```python
from build123d import *

# Parameters (mm, degrees)
SKETCH1_R               = 10
SKETCH1_W               = 40
SKETCH1_H               = 8
BOSS_EXTRUDE1_DEPTH     = 12
BOSS_EXTRUDE2_DEPTH     = 19
CUT_EXTRUDE1_DEPTH      = 38
CUT_EXTRUDE1_DEPTH_BACK = 38
SKETCH4_R               = 6
FILLET1_R               = 7
SKETCH6_R               = 6.25
CUT_EXTRUDE2_DEPTH      = 5
CUT_EXTRUDE3_DEPTH      = 56
CUT_EXTRUDE3_DEPTH_BACK = 21
SKETCH9_R               = 5
CUT_EXTRUDE4_DEPTH      = 14
SKETCH10_R              = 5
CUT_EXTRUDE5_DEPTH      = 11


with BuildPart() as part:
    # Sketch1 → Boss-Extrude1 (new, symmetric)
    # profile 1 of 2: a face of its own
    with BuildSketch(Plane.XY):
        Polygon((49.483339502, 12.718271103), (43.983339502, 22.244550544), (0, 30), (-8, 30), (-30.516660498, 17), (-30.516660498, 8), (-30.516660498, 0), (0, 0), (27.454647768, 0), align=None)
        with Locations((-4, 15)):
            Circle(SKETCH1_R, mode=Mode.SUBTRACT)
    # profile 2 of 2: a face of its own
    with BuildSketch(Plane.XY):
        with Locations((-50.516660498, 4)):
            Rectangle(SKETCH1_W, SKETCH1_H)
    extrude(amount=BOSS_EXTRUDE1_DEPTH, both=True)

    # Sketch2 → Boss-Extrude2 (add, symmetric)
    with BuildSketch(Plane.XY):
        Polygon((17.483339502, 26.917215533), (17.483339502, 0), (27.454647768, 0), (49.483339502, 12.718271103), (43.983339502, 22.244550544), align=None)
    extrude(amount=BOSS_EXTRUDE2_DEPTH, both=True)

    # Sketch4 → Cut-Extrude1 (cut, two sides: drawn at the far end of the back side and taken through both)
    with BuildSketch(Plane(origin=(1.363661942, -2.361931768, 0), x_dir=(-0.8660254037844379, -0.5000000000000014, 0), z_dir=(0.5000000000000014, -0.8660254037844379, 0)).offset(-CUT_EXTRUDE1_DEPTH_BACK)):
        with Locations((-31.137235053, 6)):
            Circle(SKETCH4_R)
        with Locations((-38.137235053, -6)):
            Circle(SKETCH4_R)
    extrude(amount=CUT_EXTRUDE1_DEPTH + CUT_EXTRUDE1_DEPTH_BACK, mode=Mode.SUBTRACT)

    # Fillet1
    fillet1_edges = [part.edges().sort_by_distance(p)[0] for p in [
        (17.483339502, 13.458607766, -12),
        (17.483339502, 13.458607766, 12),
    ]]
    fillet(fillet1_edges, radius=FILLET1_R - 0.0001)  # a hair under: the kernel refuses the full size

    # Sketch6 → Cut-Extrude2 (cut)
    with BuildSketch(Plane(origin=(0, 8, 0), x_dir=(1, 0, 0), z_dir=(0, 1, 0))):
        with Locations(Location((-61.516660498, 0, 0), (0, 0, 180))):
            Circle(SKETCH6_R)
    extrude(amount=-CUT_EXTRUDE2_DEPTH, mode=Mode.SUBTRACT)

    # Sketch8 → Cut-Extrude3 (cut, two sides: drawn at the far end of the back side and taken through both)
    with BuildSketch(Plane(origin=(0, 0, 0), x_dir=(0, 0, -1), z_dir=(1, 0, 0)).offset(-CUT_EXTRUDE3_DEPTH_BACK)):
        with BuildLine():
            Line((-9.5, 30), (-2.5, 30))
            ThreePointArc((-2.5, 30), (-6, 26.5), (-9.5, 30))
        make_face()
        with BuildLine():
            Line((2.5, 30), (9.5, 30))
            ThreePointArc((9.5, 30), (6, 26.5), (2.5, 30))
        make_face()
    extrude(amount=CUT_EXTRUDE3_DEPTH + CUT_EXTRUDE3_DEPTH_BACK, mode=Mode.SUBTRACT)

    # Sketch9 → Cut-Extrude4 (cut)
    with BuildSketch(Plane.XY.offset(19)):
        with Locations((34.148109615, 17.12820927)):
            Circle(SKETCH9_R)
    extrude(amount=-CUT_EXTRUDE4_DEPTH, mode=Mode.SUBTRACT)

    # Sketch10 → Cut-Extrude5 (cut)
    with BuildSketch(Plane(origin=(0, 0, -19), x_dir=(-1, 0, 0), z_dir=(0, 0, -1))):
        with Locations((-26.120496882, 17.032442386)):
            Circle(SKETCH10_R)
    extrude(amount=-CUT_EXTRUDE5_DEPTH, mode=Mode.SUBTRACT)


solid = part.part
```
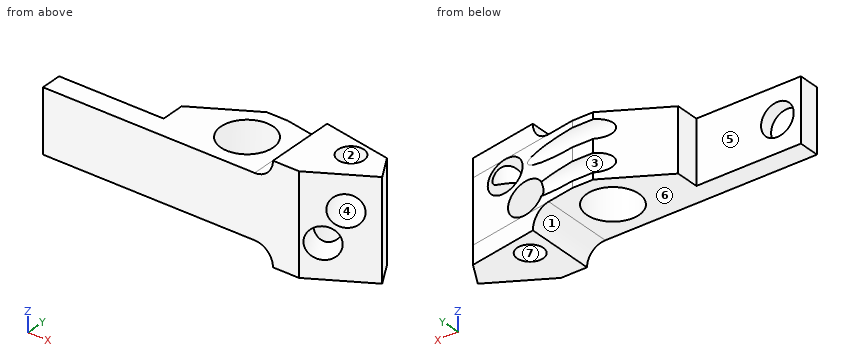
Verification items for the finished model (mm, model axes). Face numbers are marked on the shaded views. A direction names the side the tool comes from. Give positions to 0.01 mm unless a question says otherwise; leave off trailing zeros. Order: outer loops, then holes, each group sorted by start corner. A loop starts at its lowest first (then second) coordinate and runs counter-clockwise, first axis right, second up. Notation, with made-up numbers: (62.5, -36) -> (87.5, -36) arc R33 ccw to (87.5, -2) -> close; hole circle Ø5 at (-16.5, 35.5). An arc over 180 degrees is marked (long way). Use a Markdown table: item, result.
1) Mould release check, pull along Z, two halves, no side actions. Record for the marked faces 1, 2, 3 and 4: pulls with the +Z half, pulls with the -Z half, needs draft (parallel to the pull), parting line crosses it, or undercut.
Results:
| item | result |
|---|---|
| face 1 | pulls with the -Z half |
| face 2 | needs draft |
| face 3 | undercut |
| face 4 | undercut |
2) Section check C-C, the plane x = -59. Record the boundary of the cut face in (y, z).
Results:
| item | result |
|---|---|
| outline | (0, -12) -> (8, -12) -> (8, -5.72) -> (3, -5.72) -> (3, 5.72) -> (8, 5.72) -> (8, 12) -> (0, 12) -> close |
3) Depth check by flat-ended pin: pin 1 Ø12 at (x, y) = (-4, 15) entering from -Z; pin 2 Ø4 at (y, z) = (11.5, -13.5) entering from -X; pin 3 Ø9 at (x, y) = (-32, 20.5) entering from -Z; pin 4 Ø7 at (x, z) = (-56.5, 0.5) entering from +Y. Enter the tip coordinate at first touch or a pass-through.
Results:
| item | result |
|---|---|
| pin 1 | through |
| pin 2 | x = -30.52 |
| pin 3 | z = -12 |
| pin 4 | y = 8 |
4) Tool access check on the marked faces 5, 6 and 7. Record the directions out of +Z, -Z, +X, -X, +Y, -Y that give a thin tool (end or side, any length) a straight path to the whole face; none if there is none.
Results:
| item | result |
|---|---|
| face 5 | +Z, -Z, -X, +Y |
| face 6 | -Z, -X, +Y, -Y |
| face 7 | -Z |
5) Section check A-A, the plane x = -4. Record the boundary of the cut face in (y, z), then the cut area to 3 significant figures.
Results:
| item | result |
|---|---|
| outline | (0, -12) -> (5, -12) -> (5, 12) -> (0, 12) -> close; (25, -12) -> (30, -12) -> (30, -9.5) arc R3.5 cw to (30, -2.5) -> (30, 2.5) arc R3.5 cw to (30, 9.5) -> (30, 12) -> (25, 12) -> close |
| area | 202 mm² |
6) Section check B-B, the plane y = 10.5. Give the number of separate pieces and of enclosed holes in the cut face, then the cut area to 3 significant figures.
Results:
| item | result |
|---|---|
| separate pieces | 2 |
| enclosed holes | 2 |
| area | 1,550 mm² |
7) Material ranges on probe 1 along Z at (x, y) = (28, 23); probe 2 along X at (y, z) = (11.5, 3.5); probe 3 along X at (y, z) = (18, -10.5), recorded low to high.
Results:
| item | result |
|---|---|
| probe 1 | -19 to -9.84, -2.16 to 0.5, 11.5 to 19 |
| probe 2 | -30.52 to -13.37, 5.37 to 31.1, 43.7 to 47.37 |
| probe 3 | -28.78 to -13.54, 5.54 to 20.98, 31.03 to 46.43 |
